Work out the finished part from the listing and answer in its coordinate system (mm). Coordinates: 2 decimals unless noted, no trailing zeros. Order: outer loops, then holes, each group sorted by start corner. A loop starts at its lowest first (then second) coordinate and runs counter-clockwise, first axis right, second up. Notation, with made-up numbers: M -5.75,-4.75 L 51.25,-4.75 A31 ccw 51.25,28.25 Z; hole C 31,-37.5 d10. An arc over 180 degrees is marked long. Use a Markdown table: item, result.
Autodesk Inventor part; units mm, degrees
ref_plane "YZ Plane" through (0, 0, 0) normal (1, 0, 0) x (0, 1, 0)
ref_plane "XZ Plane" through (0, 0, 0) normal (0, 1, 0) x (-1, 0, 0)
ref_plane "XY Plane" through (0, 0, 0) normal (0, 0, 1) x (1, 0, 0)
sketch "Sketch3" plane through (0, 0, 0) normal (0, 1, 0) x (-1, 0, 0)
  line L0 (6.6262, -36.1747) -> (16.6262, -27.3275)
  arc A0 (16.6262, -27.3275) -> (20, -19.8379) centre (10, -19.8379) ccw
  line L1 (20, -19.8379) -> (20, -7.6759)
  arc A1 (20, -7.6759) -> (18, -1.6759) centre (10, -7.6759) ccw
  line L2 (18, -1.6759) -> (14.5, 2.9908)
  arc A2 (12.5, 8.9908) -> (14.5, 2.9908) centre (22.5, 8.9908) ccw
  arc A3 (-14.5, 2.9908) -> (-12.5, 8.9908) centre (-22.5, 8.9908) ccw
  line L3 (-14.5, 2.9908) -> (-18, -1.6759)
  arc A4 (-18, -1.6759) -> (-20, -7.6759) centre (-10, -7.6759) ccw
  line L4 (-20, -7.6759) -> (-20, -19.8379)
  arc A5 (-20, -19.8379) -> (-16.6262, -27.3275) centre (-10, -19.8379) ccw
  line L5 (-16.6262, -27.3275) -> (-6.6262, -36.1747)
  arc A6 (-6.6262, -36.1747) -> (6.6262, -36.1747) centre (0, -28.6852) ccw
  line L6 (-7.8135, -19.9641) -> (-6.7529, -18.9034)
  arc A7 (-4.5608, -21.0955) -> (-6.7529, -18.9034) centre (-5.6569, -19.9994) ccw
  line L7 (-4.5608, -21.0955) -> (-5.6215, -22.1561)
  arc A8 (-7.8135, -19.9641) -> (-5.6215, -22.1561) centre (-6.7175, -21.0601) ccw
  arc A9 (5.6215, -22.1561) -> (7.8135, -19.9641) centre (6.7175, -21.0601) ccw
  line L8 (5.6215, -22.1561) -> (4.5608, -21.0955)
  arc A10 (6.7529, -18.9034) -> (4.5608, -21.0955) centre (5.6569, -19.9994) ccw
  line L9 (6.7529, -18.9034) -> (7.8135, -19.9641)
  arc A11 (-6.7529, -9.7817) -> (-4.5608, -7.5897) centre (-5.6569, -8.6857) ccw
  line L10 (-6.7529, -9.7817) -> (-7.8135, -8.7211)
  arc A12 (-5.6215, -6.5291) -> (-7.8135, -8.7211) centre (-6.7175, -7.6251) ccw
  line L11 (-5.6215, -6.5291) -> (-4.5608, -7.5897)
  arc A13 (7.8135, -8.7211) -> (5.6215, -6.5291) centre (6.7175, -7.6251) ccw
  line L12 (7.8135, -8.7211) -> (6.7529, -9.7817)
  arc A14 (4.5608, -7.5897) -> (6.7529, -9.7817) centre (5.6569, -8.6857) ccw
  line L13 (4.5608, -7.5897) -> (5.6215, -6.5291)
  circle A15 centre (0, -14.3426) radius 3
  line L14 (-12.5, 8.9908) -> (12.5, 8.9908) construction
  arc A16 (12.5, 104.6916) -> (12.2297, 109.0328) centre (-22.5, 104.6916) ccw
  line L15 (12.2297, 109.0328) -> (10, 126.8706)
  line L16 (10, 126.8706) -> (10, 134.8706)
  arc A17 (10, 134.8706) -> (8, 136.8706) centre (8, 134.8706) ccw
  line L17 (8, 136.8706) -> (2, 136.8706)
  arc A18 (2, 136.8706) -> (0, 134.8706) centre (2, 134.8706) ccw
  line L18 (0, 134.8706) -> (0, 128.8706)
  arc A19 (-2, 126.8706) -> (0, 128.8706) centre (-2, 128.8706) ccw
  line L19 (-2, 126.8706) -> (-8.2344, 126.8706)
  arc A20 (-8.2344, 126.8706) -> (-10.219, 125.1187) centre (-8.2344, 124.8706) ccw
  line L20 (-10.219, 125.1187) -> (-12.2297, 109.0328)
  arc A21 (-12.2297, 109.0328) -> (-12.5, 104.6916) centre (22.5, 104.6916) ccw
  circle A22 centre (6, 106.8706) radius 1.5
  circle A23 centre (-6, 106.8706) radius 1.5
  circle A24 centre (0, 94.4442) radius 1.5
  circle A25 centre (0, 115.6574) radius 4
  line L21 (-12.5, 104.6916) -> (12.5, 104.6916) construction
  line L22 (0, -14.3426) -> (0, 115.6574)
  line L23 (12.5, 8.9908) -> (12.5, 104.6916)
  line L24 (-12.5, 104.6916) -> (-12.5, 8.9908)
  dimension "d4" = 21.2132
  dimension "d7" = 12
  dimension "d8" = 130
extrude "Extrusion1" add sketch "Sketch3" along normal blind 3
sketch "Sketch4" plane through (0, 3, 0) normal (0, 1, 0) x (1, 0, 0)
  circle A0 centre (0, 14.3426) radius 3 construction
  circle A1 centre (0, 14.3426) radius 88.9 construction
  circle A2 centre (0, -115.6574) radius 4
  point P0 (0, 0)
  dimension "d9" = 177.8
  dimension "d10" = 130
sketch "Sketch5" plane through (0, 3, 0) normal (0, 1, 0) x (1, 0, 0)
  line L0 (-12.5, -8.9908) -> (-12.5, -104.6916)
  line L1 (12.5, -104.6916) -> (12.5, -8.9908)
  arc A0 (-12.5, -8.9908) -> (-14.5, -2.9908) centre (-22.5, -8.9908) ccw
  arc A1 (14.5, -2.9908) -> (12.5, -8.9908) centre (22.5, -8.9908) ccw
  line L2 (14.5, -2.9908) -> (18, 1.6759)
  line L3 (-18, 1.6759) -> (-14.5, -2.9908)
  circle A2 centre (0, -94.4442) radius 1.5 construction
  line L4 (0, 0) -> (0, -94.4442) construction
  line L5 (-7.5, 0) -> (-7.5, -94.4442)
  line L6 (7.5, 0) -> (7.5, -94.4442)
  line L7 (-18, 1.6759) -> (-14.5, -2.9908)
  line L8 (-14.5, -2.9908) -> (-7.5, -12.3241)
  line L9 (14.5, -2.9908) -> (7.5, -12.3241)
  circle A3 centre (0, 14.3426) radius 88.9 construction
  line L10 (-7.5, -74.2405) -> (-12.5, -81.1047)
  line L11 (7.5, -74.2405) -> (12.5, -80.9071)
  arc A4 (-16.6262, 27.3275) -> (-20, 19.8379) centre (-10, 19.8379) ccw construction
  dimension "d11" = 7.5
  dimension "d12" = 7.5
  dimension "d13" = 143.13
  dimension "d14" = 143.13
  dimension "d15" = 143.93
  dimension "d18" = 10
extrude "Extrusion2" [suppressed]
fillet "Fillet1" [suppressed]
properties part number "Kauri arm short"
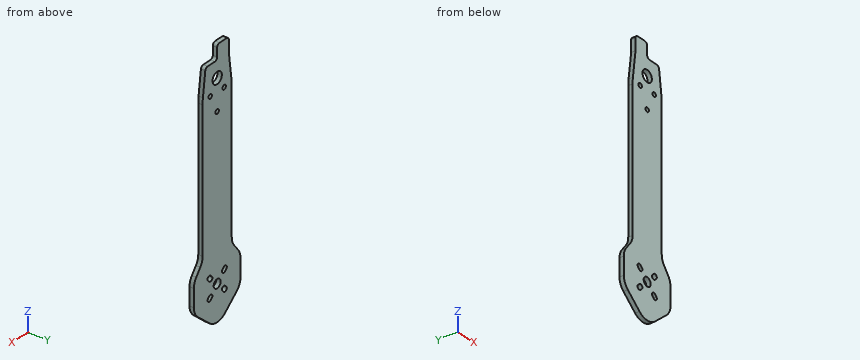
1. Find the intervals of material crossed by probe 1 along Z at (x, y) = (6, 2.1); probe 2 along Z at (x, y) = (-8, 1.5); probe 3 along X at (y, z) = (0.45, 36), in increasing order.
Answers below:
| item | result |
|---|---|
| probe 1 | -36.69 to -22.43, -18.49 to -10.2, -6.25 to 105.37, 108.37 to 126.87 |
| probe 2 | -34.96 to -21.93, -20.19 to -8.5, -6.75 to 136.87 |
| probe 3 | -12.5 to 12.5 |
2. Flat-ended cylindrical pins translate along their axes: P1, Ø3.5, axis at x = 0, z = -14.34, coming from the +Y side; P2, Ø1, axis at x = 2.5, y = 1.5, coming from the -Z side; P3, Ø1.5, axis at y = 2, z = 56.5, coming from the -X side; P4, Ø1.5, axis at y = 1.5, z = 131, coming from the -X side. Find the tip coordinate at first contact, or state that the pin passes through.
Answers below:
| item | result |
|---|---|
| P1 | through |
| P2 | z = -38.48 |
| P3 | x = -12.5 |
| P4 | x = -10 |
3. Section A-A on z = 23 is taken. Determine the outline of the cut face in (x, y).
Answers below:
| item | result |
|---|---|
| outline | M -12.5,0 L 12.5,0 L 12.5,3 L -12.5,3 Z |
4. Section B-B on y = 2.15 is taken. Give the number of separate pieces and of enclosed holes in the cut face, then the cut area to 3 significant figures.
Answers below:
| item | result |
|---|---|
| separate pieces | 1 |
| enclosed holes | 9 |
| area | 4,390 mm² |
